from build123d import *

# Parameters (mm, degrees)
SKETCH_1_W      = 60
SKETCH_1_H      = 50
SKETCH_1_R      = 1.6
SKETCH_1_R_2    = 1.1
EXTRUDE_1_DEPTH = 3
FILLET_1_R      = 2
FILLET_2_R      = 2
FILLET_3_R      = 3


with BuildPart() as part:
    # 草图1 → 凸台-拉伸1 (new body)
    with BuildSketch(Plane(origin=(0, 0, 0), x_dir=(1, 0, 0), z_dir=(0, 1, 0))):
        Rectangle(SKETCH_1_W, SKETCH_1_H)
        with Locations((-25, 21)):
            Circle(SKETCH_1_R, mode=Mode.SUBTRACT)
        with Locations((25, 21)):
            Circle(SKETCH_1_R, mode=Mode.SUBTRACT)
        with Locations((25, -21)):
            Circle(SKETCH_1_R, mode=Mode.SUBTRACT)
        with Locations((-25, -21)):
            Circle(SKETCH_1_R, mode=Mode.SUBTRACT)
        with Locations((18.6, 0)):
            Circle(SKETCH_1_R_2, mode=Mode.SUBTRACT)
        with Locations((-18.6, 8.8)):
            Circle(SKETCH_1_R_2, mode=Mode.SUBTRACT)
        with Locations((-18.6, -8.8)):
            Circle(SKETCH_1_R_2, mode=Mode.SUBTRACT)
        with BuildLine():
            Line((-25, -5.3), (-25, 5.3))
            Line((-25, 5.3), (-18.6, 5.3))
            ThreePointArc((-18.6, 5.3), (-15.1, 8.8), (-18.6, 12.3))
            Line((-18.6, 12.3), (-25, 12.3))
            Line((-25, 12.3), (-25, 17))
            ThreePointArc((-25, 17), (-23, 17.535898385), (-21.535898385, 19))
            Line((-21.535898385, 19), (21.535898385, 19))
            ThreePointArc((21.535898385, 19), (23, 17.535898385), (25, 17))
            Line((25, 17), (25, 3.5))
            Line((25, 3.5), (18.6, 3.5))
            ThreePointArc((18.6, 3.5), (15.1, 0), (18.6, -3.5))
            Line((18.6, -3.5), (25, -3.5))
            Line((25, -3.5), (25, -17))
            ThreePointArc((25, -17), (23, -17.535898385), (21.535898385, -19))
            Line((21.535898385, -19), (-21.535898385, -19))
            ThreePointArc((-21.535898385, -19), (-23, -17.535898385), (-25, -17))
            Line((-25, -17), (-25, -12.3))
            Line((-25, -12.3), (-18.6, -12.3))
            ThreePointArc((-18.6, -12.3), (-15.1, -8.8), (-18.6, -5.3))
            Line((-18.6, -5.3), (-25, -5.3))
        make_face(mode=Mode.SUBTRACT)
    extrude(amount=EXTRUDE_1_DEPTH)

    # 圆角1
    fillet_1_edges = [part.edges().sort_by_distance(p)[0] for p in [
        (30, 1.5, 25),
        (-30, 1.5, 25),
        (-30, 1.5, -25),
        (30, 1.5, -25),
    ]]
    fillet(fillet_1_edges, radius=FILLET_1_R)

    # 圆角2
    fillet_2_edges = [part.edges().sort_by_distance(p)[0] for p in [
        (-25, 1.5, 17),
        (-21.535898385, 1.5, 19),
        (21.535898385, 1.5, 19),
        (25, 1.5, 17),
        (25, 1.5, -17),
        (21.535898385, 1.5, -19),
        (-21.535898385, 1.5, -19),
        (-25, 1.5, -17),
    ]]
    fillet(fillet_2_edges, radius=FILLET_2_R)

    # 圆角3
    fillet_3_edges = [part.edges().sort_by_distance(p)[0] for p in [
        (-25, 1.5, -5.3),
        (-25, 1.5, 5.3),
        (-25, 1.5, 12.3),
        (25, 1.5, 3.5),
        (25, 1.5, -3.5),
        (-25, 1.5, -12.3),
    ]]
    fillet(fillet_3_edges, radius=FILLET_3_R)


solid = part.part
Geometry: final body of the model. Coordinates: model frame, mm. A direction names the side the tool comes from. Coordinates: 2 decimals unless noted, no trailing zeros. Loops run counter-clockwise (first coordinate to the right, second up) from the corner with the lowest first, then second, coordinate; pieces in that order, holes last. Notation, with made-up numbers: (23, -8) - (43, -8) arc R26 cw to (43, 24) - close; hole circle Ø11 at (-30, 56.5). An arc over 180 degrees is marked (long way). Put each result on its own line as item: value. Start each with the question number.
Q1. Set-up query: faces 5 (the cylindrical face through (-21.4, 1.5, 18.8)), 6 (the flat face through (-30, 1, 0)). Return all of +Z, -Z, +X, -X, +Y, -Y with unobstructed straight access to the full face (end or side cutting, diameter ignored); none if empty.
Q2. Cut plane C-C, the plane z = 8.8. Return loops of the section in (x, y), and give its area (3 significant figures).
Q3. Pull-direction query (X, two-part tool) for faces 1 (the cylindrical face through (-24.643, 1.521, 16.484)), 2 (the flat face through (0, 1, 25)), 3 (the cylindrical face through (-29.43, 1.52, 24.4)), 4 (the cylindrical face through (29.4, 1.52, -24.43)); classes: released by +X, released by -X, zero draft, split by the parting line, or undercut.
Q4. Line query: line 1 (Z direction, x = -18.6, y = 1.1); line 2 (X direction, y = 0.6, z = 0); line 3 (X direction, y = 0.9, z = -8.8). Output: solid intervals per line, ascending.
Q5. Cut plane D-D, the plane y = 2.05. Give the number of separate pieces and of enclosed holes in the cut face, and give its area (3 significant figures).
Q6. Cut plane B-B, the plane z = 21. Return loops of the section in (x, y).
Q7. Cut plane A-A, the plane x = -12.5. Return loops of the section in (y, z).
Filled sheet:
1. face 5: +Y, -Y
1. face 6: +Z, -Z, -X, +Y, -Y
2. outline: (-30, 0) - (-19.7, 0) - (-19.7, 3) - (-30, 3) - close; (-17.5, 0) - (-15.1, 0) - (-15.1, 3) - (-17.5, 3) - close; (25, 0) - (30, 0) - (30, 3) - (25, 3) - close
2. area: 53.1 mm²
3. face 1: undercut
3. face 2: zero draft
3. face 3: released by -X
3. face 4: released by +X
4. line 1: -25 to -19, -12.3 to -9.9, -7.7 to -5.3, 5.3 to 7.7, 9.9 to 12.3, 19 to 25
4. line 2: -30 to -25, 15.1 to 17.5, 19.7 to 30
4. line 3: -30 to -19.7, -17.5 to -15.1, 25 to 30
5. separate pieces: 1
5. enclosed holes: 8
5. area: 1,280 mm²
6. outline: (-30, 0) - (-26.6, 0) - (-26.6, 3) - (-30, 3) - close; (-23.4, 0) - (23.4, 0) - (23.4, 3) - (-23.4, 3) - close; (26.6, 0) - (30, 0) - (30, 3) - (26.6, 3) - close
7. outline: (0, -25) - (3, -25) - (3, -19) - (0, -19) - close; (0, 19) - (3, 19) - (3, 25) - (0, 25) - close
